Here's how the part is built. I have some questions about the finished solid (model axes, mm). Face numbers are marked on the shaded views. A direction names the side the tool comes from. Give positions to 0.01 mm unless a question says otherwise; leave off trailing zeros. Write each loop counter-clockwise with the first axis right and the second up, starting at its lowest first coordinate (ties: lowest second). Pieces come first, ordered by that corner, then holes. Notation, with made-up numbers: (43.25, 71.25) -> (69.25, 71.25) arc R22 ccw to (69.25, 78.25) -> close; hole circle Ø8 at (64.5, -11). An arc over 180 degrees is marked (long way). Put each result on its own line as item: value. Start each with the question number.
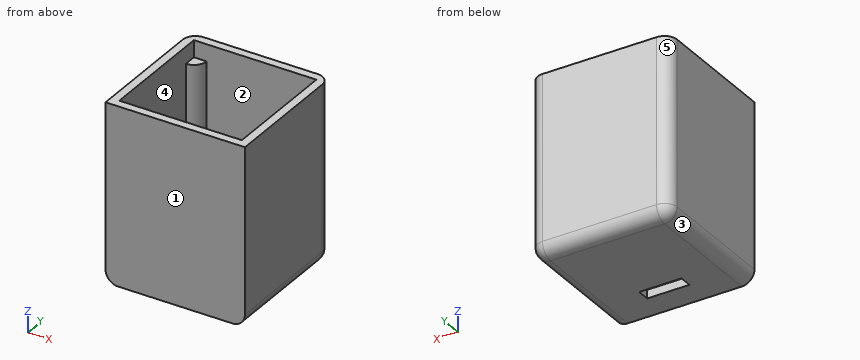
from build123d import *

# Parameters (mm, degrees)
SKETCH_1_W      = 33
SKETCH_1_H      = 32
SKETCH_1_W_2    = 29
SKETCH_1_H_2    = 28
EXTRUDE_1_DEPTH = 40
SKETCH_2_W      = 33
SKETCH_2_H      = 32
SKETCH_2_W_2    = 10
SKETCH_2_H_2    = 3
EXTRUDE_2_DEPTH = 2
EXTRUDE_3_DEPTH = 36
FILLET_1_R      = 3
FILLET_2_R      = 3
FILLET_3_R      = 3


with BuildPart() as part:
    # 草图1 → 凸台-拉伸1 (new body)
    with BuildSketch(Plane.XY):
        with Locations((0.442802767, -3.343094476)):
            Rectangle(SKETCH_1_W, SKETCH_1_H)
        with Locations((0.442802767, -3.343094476)):
            Rectangle(SKETCH_1_W_2, SKETCH_1_H_2, mode=Mode.SUBTRACT)
    extrude(amount=EXTRUDE_1_DEPTH)

    # 草图2 → 凸台-拉伸2 (add)
    with BuildSketch(Plane(origin=(0, 0, 0), x_dir=(-1, 0, 0), z_dir=(0, 0, -1))):
        with Locations((-0.442802767, -3.343094476)):
            Rectangle(SKETCH_2_W, SKETCH_2_H)
        with Locations((-0.442802767, -11.661758268)):
            Rectangle(SKETCH_2_W_2, SKETCH_2_H_2, mode=Mode.SUBTRACT)
    extrude(amount=EXTRUDE_2_DEPTH)

    # 草图5 → 凸台-拉伸3 (add)
    with BuildSketch(Plane(origin=(0, 0, 0), x_dir=(-1, 0, 0), z_dir=(0, 0, -1))):
        with BuildLine():
            Line((11.057197233, 10.656905524), (14.057197233, 10.656905524))
            Line((14.057197233, 10.656905524), (14.057197233, 7.656905524))
            ThreePointArc((14.057197233, 7.656905524), (11.935876889, 8.535585181), (11.057197233, 10.656905524))
        make_face()
        with BuildLine():
            Line((-11.942802767, 10.656905524), (-14.942802767, 10.656905524))
            Line((-14.942802767, 10.656905524), (-14.942802767, 7.656905524))
            ThreePointArc((-14.942802767, 7.656905524), (-12.821482424, 8.535585181), (-11.942802767, 10.656905524))
        make_face()
        with BuildLine():
            Line((-14.942802767, -14.343094476), (-14.942802767, -17.343094476))
            Line((-14.942802767, -17.343094476), (-11.942802767, -17.343094476))
            ThreePointArc((-11.942802767, -17.343094476), (-12.821482424, -15.221774132), (-14.942802767, -14.343094476))
        make_face()
        with BuildLine():
            Line((11.057197233, -17.343094476), (14.057197233, -17.343094476))
            Line((14.057197233, -17.343094476), (14.057197233, -14.343094476))
            ThreePointArc((14.057197233, -14.343094476), (11.935876889, -15.221774132), (11.057197233, -17.343094476))
        make_face()
    extrude(amount=-EXTRUDE_3_DEPTH)

    # 圆角1
    fillet_1_edges = [part.edges().sort_by_distance(p)[0] for p in [
        (0.442802767, 12.656905524, -2),
        (16.942802767, 12.656905524, 19),
        (-16.057197233, 12.656905524, 19),
    ]]
    fillet(fillet_1_edges, radius=FILLET_1_R)

    # 圆角2
    # the kernel refuses this fillet: 3 mm, written as the material it takes off along each edge
    with BuildSketch(Plane(origin=(13.942802767, 9.656905524, 1), x_dir=(1, 0, 0), z_dir=(0, 0, -1))) as fillet_2_piece_1_section:
        Polygon((0, 0), (FILLET_2_R, 0), (FILLET_2_R, -FILLET_2_R), (0, -FILLET_2_R), align=None)
    fillet_2_piece_1 = extrude(amount=FILLET_2_R, mode=Mode.PRIVATE)
    fillet_2_piece_1 = fillet_2_piece_1 - Plane(origin=(13.942802767, 9.656905524, 1), x_dir=(-0.7071067811865475, -0.7071067811865475, 0), z_dir=(0, 0, -1)) * Sphere(FILLET_2_R, mode=Mode.PRIVATE)
    add(fillet_2_piece_1, mode=Mode.SUBTRACT)
    with BuildSketch(Plane(origin=(16.942802767, -26.843094476, -2), x_dir=(-1, 0, 0), z_dir=(0, 1, 0))) as fillet_2_piece_2:
        with BuildLine():
            CenterArc((FILLET_2_R, FILLET_2_R), FILLET_2_R, 180, 90)
            Line((0, FILLET_2_R), (0, 0))
            Line((0, 0), (FILLET_2_R, 0))
        make_face()
    extrude(amount=36.5, mode=Mode.SUBTRACT)

    # 圆角3
    # the kernel refuses this fillet: 3 mm, written as the material it takes off along each edge
    with BuildSketch(Plane(origin=(-13.057197233, 9.656905524, 1), x_dir=(0, 0, -1), z_dir=(-1, 0, 0))) as fillet_3_piece_1_section:
        Polygon((0, 0), (FILLET_3_R, 0), (FILLET_3_R, -FILLET_3_R), (0, -FILLET_3_R), align=None)
    fillet_3_piece_1 = extrude(amount=FILLET_3_R, mode=Mode.PRIVATE)
    fillet_3_piece_1 = fillet_3_piece_1 - Plane(origin=(-13.057197233, 9.656905524, 1), x_dir=(0, -0.7071067811865475, 0.7071067811865475), z_dir=(-1, 0, 0)) * Sphere(FILLET_3_R, mode=Mode.PRIVATE)
    add(fillet_3_piece_1, mode=Mode.SUBTRACT)
    with BuildSketch(Plane(origin=(-16.057197233, 9.656905524, -2), x_dir=(0, 0, 1), z_dir=(0, -1, 0))) as fillet_3_piece_2:
        with BuildLine():
            CenterArc((FILLET_3_R, -FILLET_3_R), FILLET_3_R, 90, 90)
            Line((0, -FILLET_3_R), (0, 0))
            Line((0, 0), (FILLET_3_R, 0))
        make_face()
    extrude(amount=36.5, mode=Mode.SUBTRACT)


solid = part.part
1) I want a section at B-B, the plane z = 5. Write out the boundary of the cut face in (x, y).
2) Thinking about a two-plate mould opening in Y: for the marked faces 3, 4 and 5, which applies, released by +Y, released by -Y, zero draft, split by the parting line, or undercut?
3) I'm going to push flat-ended pins straight in: pin 1 Ø3.5 at (x, y) = (13, -15.5) entering from +Z; pin 2 Ø14 at (x, y) = (6, -2) entering from +Z; pin 3 Ø1.6 at (x, z) = (-1.5, -1.5) entering from +Y. Where does each tip first touch, or does it pass through?
4) I need wall thicknesses on probe 1 along Y at (x, z) = (5.5, 13); probe 2 along X at (y, z) = (-14, 10); probe 3 along Z at (x, y) = (-10, 3). Which ranges of each line are inside material? Lowest first, please.
5) Which directions (+Z, -Z, +X, -X, +Y, -Y) give clear straight access to the entire face, cutting with the end or side of a thin tool? Please do the marked faces 1 and 2.
6) I want a section at C-C, the plane y = -2. Write out the boundary of the cut face in (x, z).
7) I want a section at A-A, the plane x = 2.5. Write out the boundary of the cut face in (y, z), and give its area (3 significant figures).
8) I want a section at D-D, the plane x = -7. Write out the boundary of the cut face in (y, z).
Established:
1. outline: (-16.06, -19.34) -> (16.94, -19.34) -> (16.94, 9.66) arc R3 ccw to (13.94, 12.66) -> (-13.06, 12.66) arc R3 ccw to (-16.06, 9.66) -> close; hole (-14.06, -14.34) arc R3 cw to (-11.06, -17.34) -> (11.94, -17.34) arc R3 cw to (14.94, -14.34) -> (14.94, 7.66) arc R3 cw to (11.94, 10.66) -> (-11.06, 10.66) arc R3 cw to (-14.06, 7.66) -> close
2. face 3: zero draft
2. face 4: undercut
2. face 5: released by +Y
3. pin 1: stops at z = 36
3. pin 2: stops at z = 0
3. pin 3: stops at y = 12.13
4. probe 1: y = -19.34 to -17.34, 10.66 to 12.66
4. probe 2: x = -16.06 to -14.06, 14.94 to 16.94
4. probe 3: z = -2 to 0
5. face 1: +Z, -Z, +X, -X, -Y
5. face 2: +Z
6. outline: (-16.06, 1) arc R3 ccw to (-13.06, -2) -> (13.94, -2) arc R3 ccw to (16.94, 1) -> (16.94, 40) -> (14.94, 40) -> (14.94, 0) -> (-14.06, 0) -> (-14.06, 40) -> (-16.06, 40) -> close
7. outline: (-19.34, -2) -> (-13.16, -2) -> (-13.16, 0) -> (-17.34, 0) -> (-17.34, 40) -> (-19.34, 40) -> close; (-10.16, -2) -> (9.66, -2) arc R3 ccw to (12.66, 1) -> (12.66, 40) -> (10.66, 40) -> (10.66, 0) -> (-10.16, 0) -> close
7. area: 216 mm2
8. outline: (-19.34, -2) -> (9.66, -2) arc R3 ccw to (12.66, 1) -> (12.66, 40) -> (10.66, 40) -> (10.66, 0) -> (-17.34, 0) -> (-17.34, 40) -> (-19.34, 40) -> close
